For this review, take the finished solid that the model builds, in its own axes (mm). Face numbers are marked on the shaded views. Coordinates: 2 decimals unless noted, no trailing zeros. Loops run counter-clockwise (first coordinate to the right, second up) from the corner with the lowest first, then second, coordinate; pieces in that order, holes last. Notation, with made-up numbers: (14.5, -0.75) - (40.5, -0.75) arc R30 ccw to (40.5, 23.25) - close; hole circle Ø1 at (-27.75, -27). An arc over 180 degrees is marked (long way). Answer as a JSON object with one key per item and string values. Group by question number.
Item 1: To check wall thickness, follow line 1 (Z direction, x = -13, y = 0); line 2 (X direction, y = -17.5, z = -7); line 3 (Y direction, x = -14, z = 5). State the ranges of each line that lie inside material, in increasing order.
Item 2: We need section A-A (x = -9.25). Give the boundary of the cut face in (y, z).
Item 3: Clearance check with flat-ended pins moving along their axes: pin 1 (21.5 mm diameter, centred on y = 1.5, z = 8.5, fed in from +X); pin 2 (2 mm diameter, centred on x = -13.5, z = -11.5, fed in from +Y); pin 3 (5 mm diameter, centred on x = -10.5, z = 6, fed in from -Y); pin 4 (1 mm diameter, centred on x = -10.5, y = -13, fed in from -Z). State where each tip first meets the part, or that it passes through.
Item 4: Mouldability with a two-part tool opening along Y and no side actions: class the marked faces 1, 2 and 3 as released by +Y, released by -Y, zero draft, split by the parting line, or undercut.
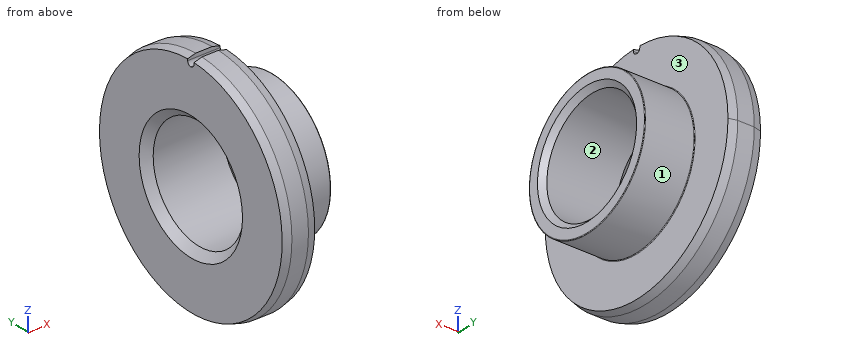
from build123d import *

# Parameters (mm, degrees)
F2_SIZE  = 1
F3_SIZE  = 1.5
F5_DEPTH = 25
F6_R     = 0.12


with BuildPart() as f1:
    # F0 (on Top) → F1 (revolve)
    with BuildSketch(Plane.XY):
        Polygon((-20.277789, 22.15), (-21.827789, 21.734679), (-21.827789, 10.8), (-5.927789, 10.8), (-5.927789, 13.8), (-15.527789, 13.8), (-15.527789, 21.734679), (-17.077789, 22.15), align=None)
    revolve(axis=Axis((-0.12533, 0, 0), (1, 0, 0)))

    # F2
    f2_edges = [f1.edges().sort_by_distance(p)[0] for p in [
        (-5.927789, -10.8, 0),
    ]]
    chamfer(f2_edges, length=F2_SIZE)

    # F3
    f3_edges = [f1.edges().sort_by_distance(p)[0] for p in [
        (-21.827789, -10.8, 0),
    ]]
    chamfer(f3_edges, length=F3_SIZE)

    # F4 (on face) → F5 (cut)
    with BuildSketch(Plane(origin=(-21.827789, 0, 0), x_dir=(0, -1, 0), z_dir=(-1, 0, 0))):
        with BuildLine():
            ThreePointArc((-0.75, 21.4), (-0.53033, 20.86967), (0, 20.65))
            Line((0, 20.65), (0, 23.059197))
            Line((0, 23.059197), (-0.75, 23.059197))
            Line((-0.75, 23.059197), (-0.75, 21.4))
        make_face()
        with BuildLine():
            Line((0, 23.059197), (0, 20.65))
            ThreePointArc((0, 20.65), (0.53033, 20.86967), (0.75, 21.4))
            Line((0.75, 21.4), (0.75, 23.059197))
            Line((0.75, 23.059197), (0, 23.059197))
        make_face()
        with BuildLine():
            ThreePointArc((0, 21.734679), (0.375056, 21.731443), (0.75, 21.721735))
            Line((0.75, 21.721735), (0.75, 23.059197))
            Line((0.75, 23.059197), (0, 23.059197))
            Line((0, 23.059197), (0, 21.734679))
        make_face()
        with BuildLine():
            Line((-0.75, 23.059197), (-0.75, 21.721735))
            ThreePointArc((-0.75, 21.721735), (-0.375056, 21.731443), (0, 21.734679))
            Line((0, 21.734679), (0, 23.059197))
            Line((0, 23.059197), (-0.75, 23.059197))
        make_face()
        with BuildLine():
            ThreePointArc((0, 21.734679), (-0.375056, 21.731443), (-0.75, 21.721735))
            Line((-0.75, 21.721735), (-0.75, 21.4))
            ThreePointArc((-0.75, 21.4), (-0.53033, 20.86967), (0, 20.65))
            Line((0, 20.65), (0, 21.734679))
        make_face()
        with BuildLine():
            Line((0.75, 21.4), (0.75, 21.721735))
            ThreePointArc((0.75, 21.721735), (0.375056, 21.731443), (0, 21.734679))
            Line((0, 21.734679), (0, 20.65))
            ThreePointArc((0, 20.65), (0.53033, 20.86967), (0.75, 21.4))
        make_face()
    extrude(amount=-F5_DEPTH, mode=Mode.SUBTRACT)

    # F6
    f6_edges = [f1.edges().sort_by_distance(p)[0] for p in [
        (-15.527789, -13.8, 0),
        (-5.927789, -13.8, 0),
    ]]
    fillet(f6_edges, radius=F6_R)


solid = f1.part
Check sheet entries:
{
 "1": {"line 1": "z = -13.8 to -10.8, 10.8 to 13.8", "line 2": "x = -21.83 to -15.53", "line 3": "y = -12.86 to -9.57, 9.57 to 12.86"},
 "2": {"outline": "circle Ø27.6 at (0, 0); hole circle Ø21.6 at (0, 0)"},
 "3": {"pin 1": "stops at x = -5.93", "pin 2": "stops at y = 8.95", "pin 3": "stops at y = -13.35", "pin 4": "stops at z = -5.85"},
 "4": {"face 1": "split by the parting line", "face 2": "undercut", "face 3": "zero draft"}
}
